Can you work these out from the model? Positions are in its coordinate system, mm. A direction names the side the tool comes from. Give positions to 0.01 mm unless a question says otherwise; leave off trailing zeros. Loops run counter-clockwise (first coordinate to the right, second up) from the corner with the lowest first, then second, coordinate; pieces in that order, holes last. Notation, with made-up numbers: M -24,44.25 L -5,44.25 A15 ccw -5,69.25 Z; hole C 73.5,-1 d7. An arc over 180 degrees is marked long. Answer as a JSON object with one key per item and string values.
```python
from build123d import *

# Parameters (mm, degrees)
SKETCH_1_W          = 75
SKETCH_1_H          = 56
EXTRUDE_1_DEPTH     = 5
SKETCH_2_R          = 2.025
CUT_EXTRUDE_1_DEPTH = 5
CUT_EXTRUDE_2_DEPTH = 5
FILLET_1_R          = 10
SKETCH_4_R          = 1.025
CUT_EXTRUDE_3_DEPTH = 21.4
CUT_EXTRUDE_4_DEPTH = 81.4
CUT_EXTRUDE_5_DEPTH = 81.4
FILLET_2_R          = 2
FILLET_3_R          = 2


with BuildPart() as part:
    # 草图1 → 凸台-拉伸1 (new body)
    with BuildSketch(Plane.XY):
        Rectangle(SKETCH_1_W, SKETCH_1_H)
    extrude(amount=EXTRUDE_1_DEPTH)

    # 草图2 → 切除-拉伸1 (cut)
    with BuildSketch(Plane(origin=(0, 0, 0), x_dir=(-1, 0, 0), z_dir=(0, 0, -1))):
        with Locations((11.44966442, -12.653381002)):
            Circle(SKETCH_2_R)
        with Locations((0, 12.603403922)):
            Circle(SKETCH_2_R)
        with Locations((-12.544580452, -12.127821306)):
            Circle(SKETCH_2_R)
    extrude(amount=-CUT_EXTRUDE_1_DEPTH, mode=Mode.SUBTRACT)

    # 草图3 → 切除-拉伸2 (cut)
    with BuildSketch(Plane(origin=(0, 0, 0), x_dir=(-1, 0, 0), z_dir=(0, 0, -1))):
        Polygon((2.578504727, 16.603403922), (13.73197178, -8), (37.5, -8), (37.5, 28), (-37.5, 28), (-37.5, -8), (-13.73197178, -8), (-2.578504727, 16.603403922), (0, 16.603403922), align=None)
    extrude(amount=-CUT_EXTRUDE_2_DEPTH, mode=Mode.SUBTRACT)

    # 圆角1
    fillet_1_edges = [part.edges().sort_by_distance(p)[0] for p in [
        (13.73197178, -8, 2.5),
        (-13.73197178, -8, 2.5),
    ]]
    fillet(fillet_1_edges, radius=FILLET_1_R)

    # 草图4 → 切除-拉伸3 (cut)
    with BuildSketch(Plane(origin=(0, 0, 0), x_dir=(-1, 0, 0), z_dir=(0, 0, -1))):
        with Locations((30, -25.5)):
            Circle(SKETCH_4_R)
        with Locations((15, -25.5)):
            Circle(SKETCH_4_R)
        with Locations((0, -25.5)):
            Circle(SKETCH_4_R)
        with Locations((-15, -25.5)):
            Circle(SKETCH_4_R)
        with Locations((-30, -25.5)):
            Circle(SKETCH_4_R)
    extrude(amount=-CUT_EXTRUDE_3_DEPTH, mode=Mode.SUBTRACT)

    # 草图5 → 切除-拉伸4 (cut)
    with BuildSketch(Plane(origin=(0, 0, 0), x_dir=(-1, 0, 0), z_dir=(0, 0, -1))):
        Polygon((-37.5, -23), (-22.5, -8), (-37.5, -8), align=None)
        Polygon((22.5, -8), (37.5, -23), (37.5, -8), align=None)
    extrude(amount=-CUT_EXTRUDE_4_DEPTH, mode=Mode.SUBTRACT)

    # 草图6 → 切除-拉伸5 (cut)
    with BuildSketch(Plane(origin=(0, 0, 0), x_dir=(-1, 0, 0), z_dir=(0, 0, -1))):
        with BuildLine():
            Line((-3, -17.5), (-3, 4.603403922))
            ThreePointArc((-3, 4.603403922), (0, 7.603403922), (3, 4.603403922))
            Line((3, 4.603403922), (3, -17.5))
            ThreePointArc((3, -17.5), (0, -20.5), (-3, -17.5))
        make_face()
    extrude(amount=-CUT_EXTRUDE_5_DEPTH, mode=Mode.SUBTRACT)

    # 圆角2
    fillet_2_edges = [part.edges().sort_by_distance(p)[0] for p in [
        (37.5, -23, 2.5),
        (-37.5, -23, 2.5),
        (37.5, -28, 2.5),
        (-37.5, -28, 2.5),
    ]]
    fillet(fillet_2_edges, radius=FILLET_2_R)

    # 圆角3
    fillet_3_edges = [part.edges().sort_by_distance(p)[0] for p in [
        (-2.578504727, 16.603403922, 2.5),
        (2.578504727, 16.603403922, 2.5),
    ]]
    fillet(fillet_3_edges, radius=FILLET_3_R)


solid = part.part
```
1) Please list where these lines run through material, in increasing order: line 1 along Y through (x, z) = (0, 1.05) (3 decimals); line 2 along X through (y, z) = (-4.5, 0.75); line 3 along X through (y, z) = (-1.5, 2.9). Write a range as from..to.
Answer list:
{"line 1": "-28..-26.525, -24.475..-20.5, 7.603..10.578, 14.628..16.603", "line 2": "-12.58..-3, 3..12.58", "line 3": "-10.79..-3, 3..10.79"}
2) Suppose I cut it at A-A, the plane x = 30. Write out the boundary of the cut face in (y, z) (3 decimals).
Answer list:
{"outline": "M -28,0 L -26.525,0 L -26.525,5 L -28,5 Z; M -24.475,0 L -15.5,0 L -15.5,5 L -24.475,5 Z"}
3) Suppose I cut it at D-D, the plane x = -24.5. Write out the boundary of the cut face in (y, z).
Answer list:
{"outline": "M -28,0 L -10,0 L -10,5 L -28,5 Z"}
4) Suppose I cut it at B-B, the plane y = -16.5. Write out the boundary of the cut face in (x, z).
Answer list:
{"outline": "M -31,0 L -3,0 L -3,5 L -31,5 Z; M 3,0 L 31,0 L 31,5 L 3,5 Z"}
5) If we mould it in two halves opening along Y, with no side actions, what happens to faces 5 (the flat face through (3, -7, 2)), 6 (the flat face through (-7.035, 6.773, 2.465)), 7 (the flat face through (37.5, -25, 2))? For each: +Y half, -Y half, draft (parallel to the pull), parting line (faces both ways), or undercut.
Answer list:
{"face 5": "undercut", "face 6": "+Y half", "face 7": "draft"}
6) Will these pins go through, and if not, where does the flat tip stop? pin 1 Ø1.5 at (y, z) = (-6, 1.5) entering from +X; pin 2 Ø0.7 at (x, z) = (-21.5, 2) entering from +Y.
Answer list:
{"pin 1": "x = 15.34", "pin 2": "y = -8"}
7) For faces 1 (the flat face through (-21, -8, 2)), 2 (the flat face through (0, 16.603, 2)), 3 (the flat face through (-3, -6, 2)), 4 (the flat face through (21, -8, 2)), which set-ups out of +Z, -Z, +X, -X, +Y, -Y let a thin tool reach every point of the face, with its end or its side?
Answer list:
{"face 1": "+Z, -Z, -X, +Y", "face 2": "+Z, -Z, +X, -X, +Y", "face 3": "+Z, -Z", "face 4": "+Z, -Z, +X, +Y"}
8) Suppose I cut it at C-C, the plane z = 2.95. Give the number of separate pieces and of enclosed holes in the cut face, and give its area (3 significant figures).
Answer list:
{"separate pieces": "1", "enclosed holes": "9", "area": "1,470 mm^2"}
